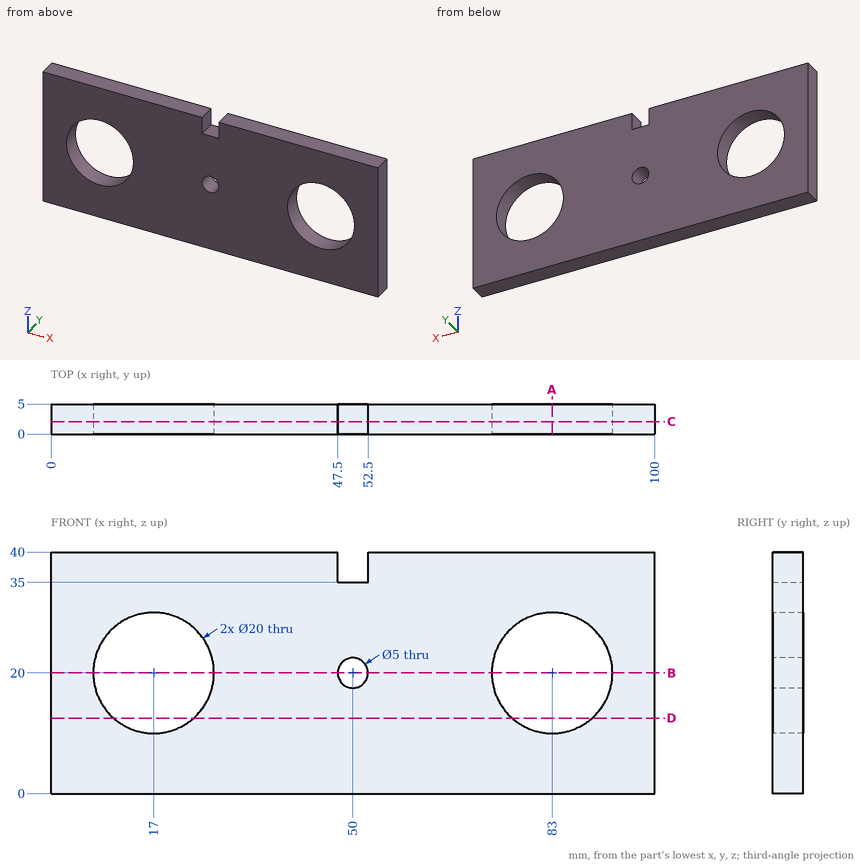
Study the drawing (mm; zero at the part's minimum x, y, z) and answer. Give positions to 0.01 mm unless a question says otherwise; leave off trailing zeros. Write each loop counter-clockwise with the first axis right and the second up, starting at its lowest first coordinate (ties: lowest second). Pieces come first, ordered by that corner, then holes.
Item 1: Section B-B, the plane z = 20 is taken. Write down the section's boundary in (x, y), plus the area to 3 significant figures.
Item 2: Section A-A, the plane x = 83 is taken. Write down the section's boundary in (y, z).
Item 3: Section D-D, the plane z = 12.5 is taken. Write down the section's boundary in (x, y).
Item 4: Find the intervals of material crossed by line 1 along Z through (x, y) = (82.5, 2.05); line 2 along X through (y, z) = (0.4, 14); line 3 along X through (y, z) = (2.5, 36), in increasing order.
Item 5: Flat-ended cylindrical pins translate along their axes: P1, Ø3, axis at y = 3.5, z = 8.5, coming from the -X side; P2, Ø2.5, axis at x = 51, y = 1.5, coming from the +Z side. Find the tip coordinate at first contact, or state that the pin passes through.
Item 6: Section C-C, the plane y = 2.1 is taken. Write down the section's boundary in (x, z).
Completed:
1. outline: (0, 0) - (7, 0) - (7, 5) - (0, 5) - close; (27, 0) - (47.5, 0) - (47.5, 5) - (27, 5) - close; (52.5, 0) - (73, 0) - (73, 5) - (52.5, 5) - close; (93, 0) - (100, 0) - (100, 5) - (93, 5) - close
1. area: 275 mm2
2. outline: (0, 0) - (5, 0) - (5, 10) - (0, 10) - close; (0, 30) - (5, 30) - (5, 40) - (0, 40) - close
3. outline: (0, 0) - (10.39, 0) - (10.39, 5) - (0, 5) - close; (23.61, 0) - (76.39, 0) - (76.39, 5) - (23.61, 5) - close; (89.61, 0) - (100, 0) - (100, 5) - (89.61, 5) - close
4. line 1: z = 0 to 10.01, 29.99 to 40
4. line 2: x = 0 to 9, 25 to 75, 91 to 100
4. line 3: x = 0 to 47.5, 52.5 to 100
5. P1: stops at x = 0
5. P2: stops at z = 35
6. outline: (0, 0) - (100, 0) - (100, 40) - (52.5, 40) - (52.5, 35) - (47.5, 35) - (47.5, 40) - (0, 40) - close; hole circle Ø20 at (17, 20); hole circle Ø5 at (50, 20); hole circle Ø20 at (83, 20)
